Input: part model. Units: mm. Frame: model coordinates. Coordinates: 2 decimals unless noted, no trailing zeros. Order: outer loops, then holes, each group sorted by start corner. A loop starts at its lowest first (then second) coordinate and runs counter-clockwise, first axis right, second up. Notation, with made-up numbers: (-11.5, 29) -> (-6.5, 29) arc R16 cw to (-6.5, 43) -> close; hole circle Ø5 at (21, 15). An arc over 180 degrees is marked (long way). One line per question, with ' | ' between items.
```python
from build123d import *

# Parameters (mm, degrees)
BOSS_EXTRUDE1_DEPTH = 2.5
SKETCH3_R           = 1
CUT_EXTRUDE1_DEPTH  = 9.5
SKETCH4_W           = 2.5
SKETCH4_H           = 2.5
BOSS_EXTRUDE3_DEPTH = 17
SKETCH5_R           = 1
CUT_EXTRUDE2_DEPTH  = 9.5


with BuildPart() as part:
    # Sketch1 → Boss-Extrude1 (new body)
    with BuildSketch(Plane.XY):
        Polygon((0, 0), (0, 1.5), (0, 2.5), (14.886845494, 2.5), (14.886845494, 1.514116192), (15.095983031, 1.72325373), (16.624293577, 0.594484955), (16.2, 0.02000738), align=None)
    extrude(amount=BOSS_EXTRUDE1_DEPTH)

    # Sketch3 → Cut-Extrude1 (cut)
    with BuildSketch(Plane.ZY):
        with Locations(Location((1.25, 1.25, 0), (0, 0, 270))):
            Circle(SKETCH3_R)
    extrude(amount=-CUT_EXTRUDE1_DEPTH, mode=Mode.SUBTRACT)

    # Sketch4 → Boss-Extrude3 (add)
    with BuildSketch(Plane.ZY):
        with Locations((1.25, 1.25)):
            Rectangle(SKETCH4_W, SKETCH4_H)
    extrude(amount=BOSS_EXTRUDE3_DEPTH)

    # Sketch5 → Cut-Extrude2 (cut)
    with BuildSketch(Plane.ZY.offset(17)):
        with Locations(Location((1.25, 1.25, 0), (0, 0, 270))):
            Circle(SKETCH5_R)
    extrude(amount=-CUT_EXTRUDE2_DEPTH, mode=Mode.SUBTRACT)


solid = part.part
```
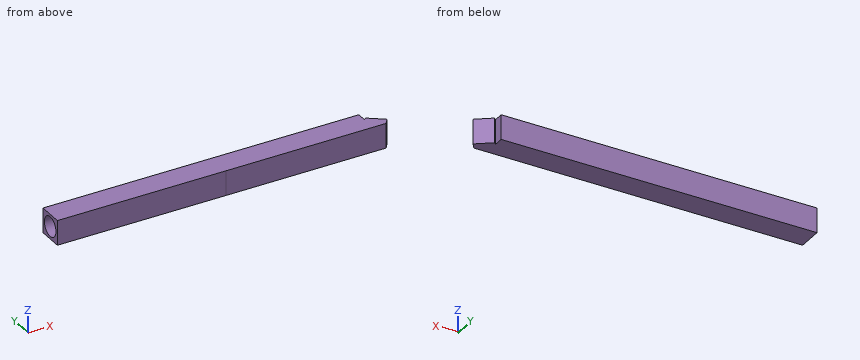
1. Pin query (flat end, axial travel): pin 1 Ø1.2 at (y, z) = (1.25, 1.25) entering from -X; pin 2 Ø1.1 at (y, z) = (2, 1) entering from +X. Return the tip coordinate at first contact, or that it passes through.
Recorded:
pin 1: stops at x = -7.5 | pin 2: stops at x = 15.47
2. Cut plane B-B, the plane x = 5. Return loops of the section in (y, z).
Recorded:
outline: (0.01, 0) -> (2.5, 0) -> (2.5, 2.5) -> (0.01, 2.5) -> close; hole circle Ø2 at (1.25, 1.25)
3. Ray query, line 1 (X direction, y = 1.8, z = 0.75); line 2 (Z direction, x = 7.25, y = 1.25); line 3 (X direction, y = 2.3, z = 2). Return the intervals inside material, ascending. Write a range as [from, to].
Recorded:
line 1: x = [-7.5, 0], [9.5, 14.89] | line 2: z = [0, 0.25], [2.25, 2.5] | line 3: x = [-17, 14.89]
4. Cut plane C-C, the plane x = 15.5. Return loops of the section in (y, z), and give its area (3 significant figures).
Recorded:
outline: (0.02, 0) -> (1.42, 0) -> (1.42, 2.5) -> (0.02, 2.5) -> close | area: 3.51 mm^2
5. Cut plane A-A, the plane z = 1.25. Return loops of the section in (x, y), and give its area (3 significant figures).
Recorded:
outline: (-17, 0) -> (0, 0) -> (16.2, 0.02) -> (16.62, 0.59) -> (15.1, 1.72) -> (14.89, 1.51) -> (14.89, 2.5) -> (-17, 2.5) -> (-17, 2.25) -> (-7.5, 2.25) -> (-7.5, 0.25) -> (-17, 0.25) -> close; hole (0, 0.25) -> (9.5, 0.25) -> (9.5, 2.25) -> (0, 2.25) -> close | area: 43.5 mm^2
